Part model, mm, in its own coordinate system. Coordinates: 2 decimals unless noted, no trailing zeros. Order: outer loops, then holes, each group sorted by start corner. A loop starts at its lowest first (then second) coordinate and runs counter-clockwise, first axis right, second up. Notation, with made-up numbers: (35.25, 34) - (60.25, 34) arc R31 ccw to (60.25, 69) - close; hole circle Ø5 at (86, 4.5). An arc over 180 degrees is marked (long way). Use a Markdown table: item, result. Add a question column.
1) Saw through at C-C on z = 141. List the corners of the cut face in (x, y), then the cut area to 3 significant figures.
2) Wall check: L1, parallel to Y at x = 0, z = 151.5; L2, parallel to Z at x = -2.25, y = -1.7; L3, parallel to X at y = 0.2, z = 106. Give the ranges that are in metal, low to high. Write a range as [from, to].
3) Drop flat-ended pins along their axis: P1, Ø1.4, axis at x = 0, y = 0, coming from the -Z side; P2, Ø1.9, axis at x = 0, y = 0, coming from the +Z side; P3, Ø3, axis at y = -2, z = 76.5, coming from the +X side. Give the stop position or say it passes through.
4) Saw through at A-A on y = 0. List the corners of the cut face in (x, z).
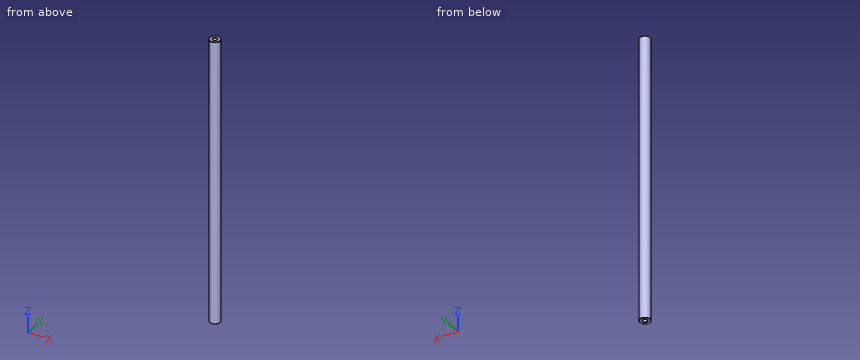
```python
from build123d import *

# Parameters (mm, degrees)
SKETCH1_R           = 3
BOSS_EXTRUDE1_DEPTH = 160
SKETCH2_R           = 1.2
CUT_EXTRUDE1_DEPTH  = 12
SKETCH3_R           = 1.2
CUT_EXTRUDE2_DEPTH  = 12
CHAMFER1_SIZE       = 0.2


with BuildPart() as part:
    # Sketch1 → Boss-Extrude1 (new body)
    with BuildSketch(Plane.XY):
        Circle(SKETCH1_R)
    extrude(amount=BOSS_EXTRUDE1_DEPTH)

    # Sketch2 → Cut-Extrude1 (cut)
    with BuildSketch(Plane.XY.offset(160)):
        Circle(SKETCH2_R)
    extrude(amount=-CUT_EXTRUDE1_DEPTH, mode=Mode.SUBTRACT)

    # Sketch3 → Cut-Extrude2 (cut)
    with BuildSketch(Plane(origin=(0, 0, 0), x_dir=(-1, 0, 0), z_dir=(0, 0, -1))):
        Circle(SKETCH3_R)
    extrude(amount=-CUT_EXTRUDE2_DEPTH, mode=Mode.SUBTRACT)

    # Chamfer1
    chamfer1_edges = [part.edges().sort_by_distance(p)[0] for p in [
        (1.2, 0, 0),
        (-3, 0, 0),
        (-3, 0, 160),
        (-1.2, 0, 160),
    ]]
    chamfer(chamfer1_edges, length=CHAMFER1_SIZE)


solid = part.part
```
Results are:
| question | item | result |
|---|---|---|
| 1 | outline | circle Ø6 at (0, 0) |
| 1 | area | 28.3 mm2 |
| 2 | L1 | [-3, -1.2], [1.2, 3] |
| 2 | L2 | [0.02, 159.98] |
| 2 | L3 | [-2.99, 2.99] |
| 3 | P1 | z = 12 |
| 3 | P2 | z = 148 |
| 3 | P3 | x = 2.96 |
| 4 | outline | (-3, 0.2) - (-2.8, 0) - (-1.4, 0) - (-1.2, 0.2) - (-1.2, 12) - (1.2, 12) - (1.2, 0.2) - (1.4, 0) - (2.8, 0) - (3, 0.2) - (3, 159.8) - (2.8, 160) - (1.4, 160) - (1.2, 159.8) - (1.2, 148) - (-1.2, 148) - (-1.2, 159.8) - (-1.4, 160) - (-2.8, 160) - (-3, 159.8) - close |
